Geometry check sheet. Reference: drawing and pictorial views, mm from the part's lowest x, y, z. A direction names the side the tool comes from. Give positions to 0.01 mm unless a question says otherwise; leave off trailing zeros. Order: outer loops, then holes, each group sorted by start corner. A loop starts at its lowest first (then second) coordinate and runs counter-clockwise, first axis right, second up.
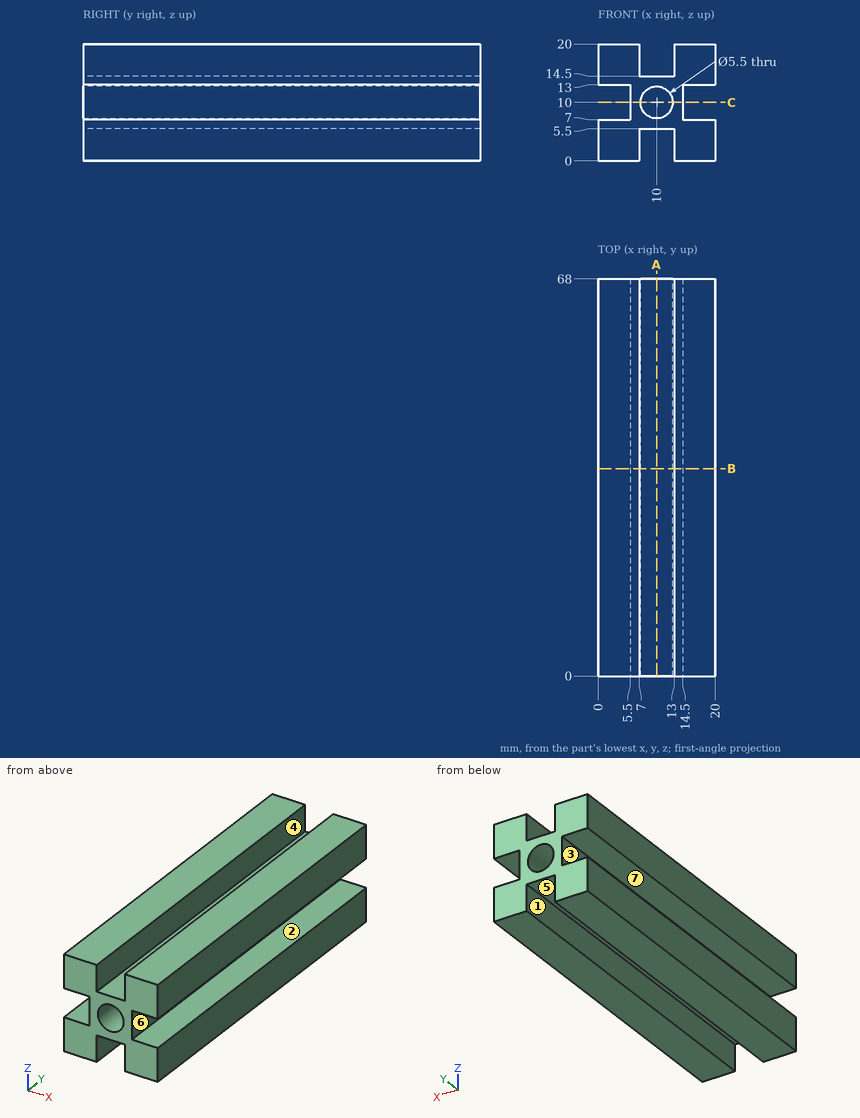
(1) Cross-section at B-B on y = 35.5. Enter the section's corners in (x, z).
Response values:
outline: (0, 0) - (7, 0) - (7, 5.5) - (13, 5.5) - (13, 0) - (20, 0) - (20, 7) - (14.5, 7) - (14.5, 13) - (20, 13) - (20, 20) - (13, 20) - (13, 14.5) - (7, 14.5) - (7, 20) - (0, 20) - (0, 13) - (5.5, 13) - (5.5, 7) - (0, 7) - close; hole circle Ø5.5 at (10, 10)
(2) Release check for a two-part mould opening along X. For the marked faces 1, 2 and 3 record: released by +X, released by -X, zero draft, split by the parting line, or undercut.
Response values:
face 1: undercut
face 2: zero draft
face 3: released by -X
(3) Gauge pin test, flat ends, axial feed: pin 1 Ø3 at (y, z) = (40.5, 11) entering from -X; pin 2 Ø1.5 at (y, z) = (33.5, 9) entering from +X; pin 3 Ø5 at (x, y) = (10, 20.5) entering from -Z. Record the tip position at first contact, or that the pin passes through.
Response values:
pin 1: stops at x = 5.5
pin 2: stops at x = 14.5
pin 3: stops at z = 5.5
(4) Material ranges on L1, parallel to X at y = 38, z = 10; L2, parallel to Z at x = 1.25, y = 5; L3, parallel to Z at x = 7.5, y = 25, recorded low to high.
Response values:
L1: x = 5.5 to 7.25, 12.75 to 14.5
L2: z = 0 to 7, 13 to 20
L3: z = 5.5 to 8.85, 11.15 to 14.5
(5) Set-up check for the marked faces 4, 5, 6 and 7: record each of +Z, -Z, +X, -X, +Y, -Y from which the full face is reachable in a straight line by a thin tool's end or side.
Response values:
face 4: +Z, +Y, -Y
face 5: -Z, +Y, -Y
face 6: +X, +Y, -Y
face 7: -X, +Y, -Y
(6) Cross-section at A-A on x = 10. Enter the section's corners in (y, z), then the cut area to 3 significant figures.
Response values:
outline: (0, 5.5) - (68, 5.5) - (68, 7.25) - (0, 7.25) - close; (0, 12.75) - (68, 12.75) - (68, 14.5) - (0, 14.5) - close
area: 238 mm2
(7) Cross-section at C-C on z = 10. Enter the section's corners in (x, y), then the cut area to 3 significant figures.
Response values:
outline: (5.5, 0) - (7.25, 0) - (7.25, 68) - (5.5, 68) - close; (12.75, 0) - (14.5, 0) - (14.5, 68) - (12.75, 68) - close
area: 238 mm2
